from build123d import *

# Parameters (mm, degrees)
F0_R      = 15
F1_DEPTH  = 10
F2_R      = 15
F3_DEPTH  = 4.5
F4_SIZE2  = 4.5
F4_SIZE   = 4.5
F5_R      = 2.2485105192
F6_DEPTH  = 4.5
F7_R      = 3.5
F8_DEPTH  = 10
F9_R      = 4.75
F9_R_2    = 2.2485105192
F10_DEPTH = 4


with BuildPart() as f1:
    # F0 (on Top) → F1 (new body)
    with BuildSketch(Plane.XY):
        Circle(F0_R)
    extrude(amount=F1_DEPTH)

    # F2 (on face) → F3 (join)
    with BuildSketch(Plane.XY.offset(10)):
        Circle(F2_R)
    extrude(amount=F3_DEPTH)

    # F4
    f4_edges = [f1.edges().sort_by_distance(p)[0] for p in [
        (-15, 0, 14.5),
    ]]
    chamfer(f4_edges, length=F4_SIZE, length2=F4_SIZE2)

    # F5 (on face) → F6 (cut)
    with BuildSketch(Plane.XY.offset(14.5)):
        Circle(F5_R)
    extrude(amount=-F6_DEPTH, mode=Mode.SUBTRACT)

    # F7 (on face) → F8 (cut)
    with BuildSketch(Plane.XY):
        Circle(F7_R)
    extrude(amount=F8_DEPTH, mode=Mode.SUBTRACT)

    # F9 (on face) → F10 (join)
    with BuildSketch(Plane.XY.offset(14.5)):
        Circle(F9_R)
        Circle(F9_R_2, mode=Mode.SUBTRACT)
    extrude(amount=F10_DEPTH)


solid = f1.part
Build history of the part. All positions in model axes, mm. A direction names the side the tool comes from. Round coordinates to 2 decimals unless told otherwise and drop trailing zeros. Write each loop counter-clockwise with the first axis right and the second up, starting at its lowest first coordinate (ties: lowest second). Pieces come first, ordered by that corner, then holes. Notation, with made-up numbers: M -28,-0.75 L 14,-0.75 A11 ccw 14,6.25 Z; hole C 77,-18 d4. An arc over 180 degrees is marked long. Answer in a Markdown table with one row per item.
1. Saw through at A-A (x = 0). List the corners of the cut face in (y, z), and give its area (3 significant figures).
Geometry check:
| item | result |
|---|---|
| outline | M -15,0 L -3.5,0 L -3.5,10 L -2.25,10 L -2.25,18.5 L -4.75,18.5 L -4.75,14.5 L -10.5,14.5 L -15,10 Z; M 2.25,10 L 3.5,10 L 3.5,0 L 15,0 L 15,10 L 10.5,14.5 L 4.75,14.5 L 4.75,18.5 L 2.25,18.5 Z |
| area | 345 mm2 |
2. Which spindle directions (+Z, -Z, +X, -X, +Y, -Y) get a long thin tool onto all of the face, cutting with end or side? Do faces 1 (the face through (2.192, -4.214, 16.472)), 2 (the face through (-2.2, -1, 18.5)). Say none if no direction does.
Geometry check:
| item | result |
|---|---|
| face 1 | +Z |
| face 2 | +Z, +X, -X, +Y, -Y |
3. Saw through at D-D (z = 15.75). List the corners of the cut face in (x, y), and give its area (3 significant figures).
Geometry check:
| item | result |
|---|---|
| outline | C 0,0 d9.5; hole C 0,0 d4.5 |
| area | 55.0 mm2 |
4. Saw through at C-C (z = 1.75). List the corners of the cut face in (x, y).
Geometry check:
| item | result |
|---|---|
| outline | C 0,0 d30; hole C 0,0 d7 |
5. Mould opens along X. For faces 3 (the face through (3.233, -1.341, 4.93)), 4 (the face through (5, -2, 14.5)), 5 (the face through (5.76, 9.04, 14.28)), 6 (the face through (0.7, -2.3, 10)) say: +X half, -X half, draft (parallel to the pull), parting line (faces both ways), or undercut.
Geometry check:
| item | result |
|---|---|
| face 3 | undercut |
| face 4 | draft |
| face 5 | parting line |
| face 6 | undercut |
6. Flat gauge pins, fed straight in: P1, Ø5, axis at y = -3, z = 7, coming from the -X side; P2, Ø6, axis at y = 8.5, z = 11.5, coming from the -X side; P3, Ø10, axis at x = -11, z = 9.5, coming from the -Y side. Where does each tip first touch, or does it go through?
Geometry check:
| item | result |
|---|---|
| P1 | x = -14.99 |
| P2 | x = -13.79 |
| P3 | y = -13.75 |
7. Probe L1, parallel to Y at x = 0, z = 5.5; L2, parallel to Z at x = 8.25, y = 1.25; L3, parallel to Y at x = 0, z = 14. List the from-to ranges inside material, lowest first. Write a range as [from, to].
Geometry check:
| item | result |
|---|---|
| L1 | [-15, -3.5], [3.5, 15] |
| L2 | [0, 14.5] |
| L3 | [-11, -2.25], [2.25, 11] |
